Model file for the job. Use its own axes, mm. Coordinates: 2 decimals unless noted, no trailing zeros. Loops run counter-clockwise (first coordinate to the right, second up) from the corner with the lowest first, then second, coordinate; pieces in that order, holes last. Notation, with made-up numbers: (-33.5, -18) -> (14.5, -18) arc R23 ccw to (14.5, -4) -> close; hole circle Ø9 at (-34.75, -9). An arc over 180 degrees is marked (long way). Use one line per item in the form item = value.
```python
from build123d import *

# Parameters (mm, degrees)
F1_DEPTH = 2.54
F3_DEPTH = 2.54
F4_R     = 0.63499


# Not quite as in the source:
# - a fillet or chamfer is up to 0.001 mm smaller than in the source, because OpenCascade refuses the exact size


with BuildPart() as f1:
    # F0 (on Top) → F1 (new body)
    with BuildSketch(Plane.XY):
        with BuildLine():
            ThreePointArc((-15.8749996872, -27.4963067508), (15.8750001564, -27.4963064799), (31.75, 0))
            ThreePointArc((31.75, 0), (15.8749996133, 27.4963067934), (-15.8750007733, 27.4963061237))
            ThreePointArc((-15.8750007733, 27.4963061237), (-31.75, -6.271e-07), (-15.8749996872, -27.4963067508))
        make_face()
        with BuildLine():
            Line((31.75, -54.9926131403), (31.75, 0))
            ThreePointArc((31.75, 0), (15.8750001564, -27.4963064799), (-15.8749996872, -27.4963067508))
            Line((-15.8749996872, -27.4963067508), (31.75, -54.9926131403))
        make_face()
        with BuildLine():
            ThreePointArc((-15.8750007733, 27.4963061237), (15.8749996133, 27.4963067934), (31.75, 0))
            Line((31.75, 0), (31.75, 54.9926131403))
            Line((31.75, 54.9926131403), (-15.8750007733, 27.4963061237))
        make_face()
        with BuildLine():
            ThreePointArc((-15.8749996872, -27.4963067508), (-31.75, -6.271e-07), (-15.8750007733, 27.4963061237))
            Line((-15.8750007733, 27.4963061237), (-63.5, 0))
            Line((-63.5, 0), (-15.8749996872, -27.4963067508))
        make_face()
    extrude(amount=F1_DEPTH)

    # F2 (on face) → F3 (join)
    with BuildSketch(Plane.XY.offset(2.54)):
        Polygon((31.75, 54.9926131403), (-63.5, 0), (31.75, -54.9926131403), align=None)
        Polygon((30.48, -52.7929086147), (-60.96, 0), (30.48, 52.7929086147), align=None, mode=Mode.SUBTRACT)
        Polygon((27.94, 48.3934995635), (-55.88, 0), (27.94, -48.3934995635), align=None)
        Polygon((-53.34, 0), (26.67, 46.1937950379), (26.67, -46.1937950379), align=None, mode=Mode.SUBTRACT)
        Polygon((24.13, 41.7943859866), (-48.26, 0), (24.13, -41.7943859866), align=None)
        Polygon((22.86, -39.594681461), (-45.72, 0), (22.86, 39.594681461), align=None, mode=Mode.SUBTRACT)
        Polygon((20.32, 35.1952724098), (-40.64, 0), (20.32, -35.1952724098), align=None)
        Polygon((19.05, -32.9955678842), (-38.1, 0), (19.05, 32.9955678842), align=None, mode=Mode.SUBTRACT)
        Polygon((16.51, 28.596158833), (-33.02, 0), (16.51, -28.596158833), align=None)
        Polygon((15.24, -26.3964543073), (-30.48, 0), (15.24, 26.3964543073), align=None, mode=Mode.SUBTRACT)
        Polygon((12.7, 21.9970452561), (-25.4, 0), (12.7, -21.9970452561), align=None)
        Polygon((-22.86, 0), (11.43, 19.7973407305), (11.43, -19.7973407305), align=None, mode=Mode.SUBTRACT)
        Polygon((8.89, -15.3979316793), (8.89, 15.3979316793), (-17.78, 0), align=None)
        Polygon((-15.24, 0), (7.62, 13.1982271537), (7.62, -13.1982271537), align=None, mode=Mode.SUBTRACT)
        Polygon((5.08, -8.7988181024), (5.08, 8.7988181024), (-10.16, 0), align=None)
        Polygon((3.81, -6.5991135768), (-7.62, 0), (3.81, 6.5991135768), align=None, mode=Mode.SUBTRACT)
        Polygon((1.27, 2.1997045256), (-2.54, 0), (1.27, -2.1997045256), align=None)
    extrude(amount=F3_DEPTH)

    # F4 (radius 0.635 in the source; OpenCascade refuses exactly that, so slightly less here)
    f4_edges = [f1.edges().sort_by_distance(p)[0] for p in [
        (-15.875, 27.496307, 5.08),
        (-15.875, -27.496307, 5.08),
        (31.75, 0, 5.08),
        (-15.24, -26.396454, 5.08),
        (-15.24, 26.396454, 5.08),
        (30.48, 0, 5.08),
        (-15.24, -26.396454, 2.54),
        (-15.24, 26.396454, 2.54),
        (30.48, 0, 2.54),
        (27.94, 0, 2.54),
        (-13.97, 24.19675, 2.54),
        (-13.97, -24.19675, 2.54),
        (27.94, 0, 5.08),
        (-13.97, 24.19675, 5.08),
        (-13.97, -24.19675, 5.08),
        (-13.335, -23.096898, 5.08),
        (-13.335, 23.096898, 5.08),
        (26.67, 0, 5.08),
        (-13.335, -23.096898, 2.54),
        (-13.335, 23.096898, 2.54),
        (26.67, 0, 2.54),
        (24.13, 0, 2.54),
        (-12.065, 20.897193, 2.54),
        (-12.065, -20.897193, 2.54),
        (24.13, 0, 5.08),
        (-12.065, 20.897193, 5.08),
        (-12.065, -20.897193, 5.08),
        (-11.43, -19.797341, 5.08),
        (-11.43, 19.797341, 5.08),
        (22.86, 0, 5.08),
        (-11.43, -19.797341, 2.54),
        (-11.43, 19.797341, 2.54),
        (22.86, 0, 2.54),
        (20.32, 0, 2.54),
        (-10.16, 17.597636, 2.54),
        (-10.16, -17.597636, 2.54),
        (20.32, 0, 5.08),
        (-10.16, 17.597636, 5.08),
        (-10.16, -17.597636, 5.08),
        (-9.525, -16.497784, 5.08),
        (-9.525, 16.497784, 5.08),
        (19.05, 0, 5.08),
        (-9.525, -16.497784, 2.54),
        (-9.525, 16.497784, 2.54),
        (19.05, 0, 2.54),
        (-8.255, 14.298079, 2.54),
        (-8.255, -14.298079, 2.54),
        (16.51, 0, 2.54),
        (-8.255, 14.298079, 5.08),
        (-8.255, -14.298079, 5.08),
        (16.51, 0, 5.08),
        (-7.62, -13.198227, 5.08),
        (-7.62, 13.198227, 5.08),
        (15.24, 0, 5.08),
        (-7.62, -13.198227, 2.54),
        (-7.62, 13.198227, 2.54),
        (15.24, 0, 2.54),
        (-6.35, 10.998523, 2.54),
        (-6.35, -10.998523, 2.54),
        (12.7, 0, 2.54),
        (-6.35, 10.998523, 5.08),
        (-6.35, -10.998523, 5.08),
        (12.7, 0, 5.08),
        (-5.715, -9.89867, 5.08),
        (-5.715, 9.89867, 5.08),
        (11.43, 0, 5.08),
        (-5.715, -9.89867, 2.54),
        (-5.715, 9.89867, 2.54),
        (11.43, 0, 2.54),
        (8.89, 0, 2.54),
        (-4.445, 7.698966, 2.54),
        (-4.445, -7.698966, 2.54),
        (8.89, 0, 5.08),
        (-4.445, 7.698966, 5.08),
        (-4.445, -7.698966, 5.08),
        (-3.81, -6.599114, 5.08),
        (-3.81, 6.599114, 5.08),
        (7.62, 0, 5.08),
        (-3.81, -6.599114, 2.54),
        (-3.81, 6.599114, 2.54),
        (7.62, 0, 2.54),
        (5.08, 0, 2.54),
        (-2.54, 4.399409, 2.54),
        (-2.54, -4.399409, 2.54),
        (5.08, 0, 5.08),
        (-2.54, 4.399409, 5.08),
        (-2.54, -4.399409, 5.08),
        (-1.905, -3.299557, 5.08),
        (-1.905, 3.299557, 5.08),
        (3.81, 0, 5.08),
        (-1.905, -3.299557, 2.54),
        (-1.905, 3.299557, 2.54),
        (3.81, 0, 2.54),
        (1.27, 0, 2.54),
        (-0.635, 1.099852, 2.54),
        (-0.635, -1.099852, 2.54),
        (1.27, 0, 5.08),
        (-0.635, 1.099852, 5.08),
        (-0.635, -1.099852, 5.08),
    ]]
    fillet(f4_edges, radius=F4_R)


solid = f1.part
```
Q1. Band-saw the part on A-A, the plane z = 0.85. Write the cut outline in (x, y), and give its area (3 significant figures).
Result:
outline = (-63.5, 0) -> (31.75, -54.99) -> (31.75, 54.99) -> close
area = 5,240 mm2
Q2. Wall check: line 1 along X through (y, z) = (-46.5, 4.45); line 2 along X through (y, z) = (40.5, 2.9); line 3 along X through (y, z) = (37.5, 3.7). Give the ranges that are in metal, low to high.
Result:
line_1 = 17.04 to 19.58, 24.66 to 27.94, 30.48 to 31.75
line_2 = 6.65 to 9.31, 14.14 to 16.93, 21.76 to 24.19, 26.61 to 28, 30.42 to 31.75
line_3 = 1.45 to 3.99, 9.07 to 11.61, 16.69 to 19.23, 22.86 to 24.13, 26.67 to 27.94, 30.48 to 31.75
Q3. Mould opens along Y. For faces 1 (the face through (-7.908, 14.498, 3.801)), 2 (the face through (-9.12, -16.73, 3.8)), 3 (the face through (-15.12, -27.72, 4.89)) say: released by +Y, released by -Y, zero draft, split by the parting line, or undercut.
Result:
face_1 = undercut
face_2 = undercut
face_3 = released by -Y
Q4. Pin check, flat tips, straight feed: pin 1 Ø8 at (x, y) = (1, -14.5) entering from -Z; pin 2 Ø1.4 at (y, z) = (-1, 4) entering from -X; pin 3 Ø1.4 at (y, z) = (-12, 3.5) entering from -X; pin 4 Ø1 at (y, z) = (-5.5, 4) entering from -X. Stop position of each tip, or through.
Result:
pin_1 = 0
pin_2 = -62.98
pin_3 = -43.93
pin_4 = -54.84
